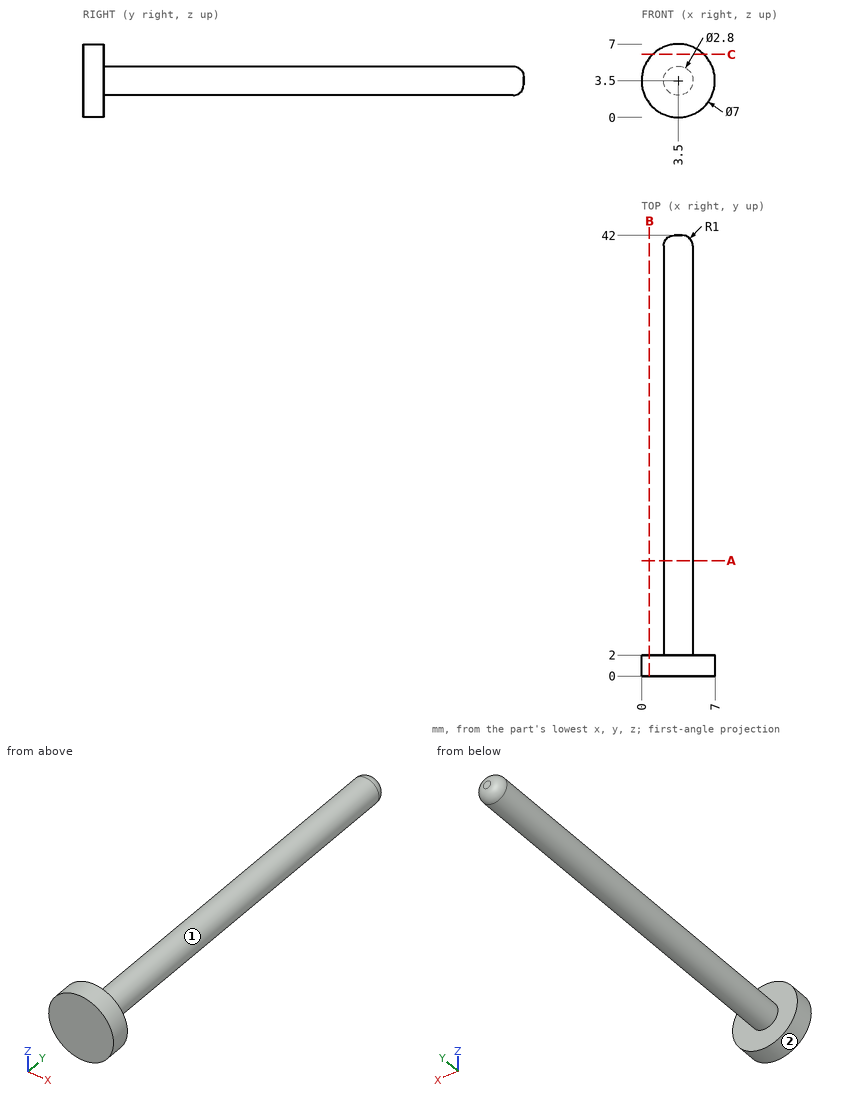
Here's the drawing with two shaded views (mm, measured from the low corner). I have some questions. A direction names the side the tool comes from. Round coordinates to 2 decimals unless told otherwise and drop trailing zeros. Write each loop counter-clockwise with the first axis right and the second up, starting at its lowest first coordinate (ties: lowest second). Pieces come first, ordered by that corner, then holes.
(1) Suppose I cut it at B-B on x = 0.75. Write out the boundary of the cut face in (y, z), and give its area (3 significant figures).
Findings below:
outline: (0, 1.33) - (2, 1.33) - (2, 5.67) - (0, 5.67) - close
area: 8.66 mm2
(2) For pin 1 (3 mm diameter, centred on x = 5.5, y = 38, fed in from +Z); pin 2 (4 mm diameter, centred on x = 4.5, z = 1, fed in from +Y), each with a flat end and sliding along its axis, tell me the tip position at first contact or that it passes through.
Findings below:
pin 1: stops at z = 4.81
pin 2: stops at y = 41.96
(3) If I drill on probe 1 along Y at (x, z) = (2.75, 5.5); probe 2 along X at (y, z) = (37.5, 4.75); probe 3 along X at (y, z) = (15, 2.5), over which ranges is the centre line in solid material (lowest first)?
Findings below:
probe 1: y = 0 to 2
probe 2: x = 2.87 to 4.13
probe 3: x = 2.52 to 4.48
(4) Suppose I cut it at C-C on z = 6. Write out the boundary of the cut face in (x, y), and give its area (3 significant figures).
Findings below:
outline: (1.05, 0) - (5.95, 0) - (5.95, 2) - (1.05, 2) - close
area: 9.80 mm2
(5) Which directions (+Z, -Z, +X, -X, +Y, -Y) give clear straight access to the entire face, cutting with the end or side of a thin tool? Please do the marked faces 1 and 2.
Findings below:
face 1: +Y
face 2: +Y, -Y
(6) Suppose I cut it at A-A on y = 11. Write out the boundary of the cut face in (x, z).
Findings below:
outline: circle Ø2.8 at (3.5, 3.5)
